Work out the finished part from the listing and answer in its coordinate system (mm). Face numbers are marked on the shaded views. A direction names the side the tool comes from. Round coordinates to 2 decimals unless told otherwise and drop trailing zeros. Loops run counter-clockwise (first coordinate to the right, second up) from the corner with the lowest first, then second, coordinate; pieces in that order, holes last. Notation, with made-up numbers: (58, -7.75) - (74, -7.75) arc R31 ccw to (74, 20.25) - close; hole circle Ø7 at (75, 38). An arc over 180 degrees is marked (long way). Use CSV: the item, a comma, the result in double quotes. Start each with the question number.
from build123d import *

# Parameters (mm, degrees)
F1_DEPTH = 20.32
F3_DEPTH = 15.24
F5_DEPTH = 25.4
F6_DEPTH = 3.175


with BuildPart() as f1:
    # F0 (on Front) → F1 (new body)
    with BuildSketch(Plane.XZ):
        Polygon((0, 31.623), (0, 0), (37.719, 0), (37.719, 3.175), (6.0198, 3.175), (6.0198, 31.623), align=None)
    extrude(amount=F1_DEPTH)

    # F2 (on face) → F3 (cut)
    with BuildSketch(Plane(origin=(0, 0, 0), x_dir=(1, 0, 0), z_dir=(0, 0, -1))):
        with BuildLine():
            Line((22.479, 6.858), (30.099, 6.858))
            ThreePointArc((30.099, 6.858), (33.401, 10.16), (30.099, 13.462))
            Line((30.099, 13.462), (22.479, 13.462))
            ThreePointArc((22.479, 13.462), (19.177, 10.16), (22.479, 6.858))
        make_face()
    extrude(amount=-F3_DEPTH, mode=Mode.SUBTRACT)

    # F4 (on face) → F5 (cut)
    with BuildSketch(Plane(origin=(0, 0, 0), x_dir=(0, -1, 0), z_dir=(-1, 0, 0))):
        with BuildLine():
            Line((13.462, 12.573), (13.462, 25.273))
            ThreePointArc((13.462, 25.273), (10.16, 28.575), (6.858, 25.273))
            Line((6.858, 25.273), (6.858, 12.573))
            ThreePointArc((6.858, 12.573), (10.16, 9.271), (13.462, 12.573))
        make_face()
    extrude(amount=-F5_DEPTH, mode=Mode.SUBTRACT)

    # F4 (on face) → F6 (cut)
    with BuildSketch(Plane(origin=(0, 0, 0), x_dir=(0, -1, 0), z_dir=(-1, 0, 0))):
        with BuildLine():
            Line((15.24, 12.573), (15.24, 25.273))
            ThreePointArc((15.24, 25.273), (10.16, 30.353), (5.08, 25.273))
            Line((5.08, 25.273), (5.08, 12.573))
            ThreePointArc((5.08, 12.573), (10.16, 7.493), (15.24, 12.573))
        make_face()
        with BuildLine():
            ThreePointArc((6.858, 25.273), (10.16, 28.575), (13.462, 25.273))
            Line((13.462, 25.273), (13.462, 12.573))
            ThreePointArc((13.462, 12.573), (10.16, 9.271), (6.858, 12.573))
            Line((6.858, 12.573), (6.858, 25.273))
        make_face(mode=Mode.SUBTRACT)
    extrude(amount=-F6_DEPTH, mode=Mode.SUBTRACT)


solid = f1.part
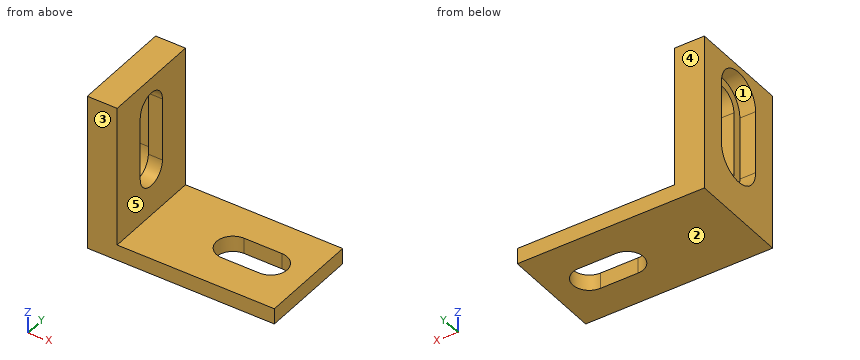
Item 1: Each of these flat-tipped pins is pushed along its axis until it touches: pin 1 Ø8 at (y, z) = (-9.5, 22.5) entering from +X; pin 2 Ø8 at (x, y) = (31, -12.5) entering from +Z (3 decimals). Where does it stop, or does it pass through?
Item 2: Find the intervals of material crossed by probe 1 along Y at (x, z) = (22.5, 3); probe 2 along Z at (x, y) = (15.5, -15.5) (3 decimals); probe 3 along X at (y, z) = (-5, 10), in increasing order. Write a range as [from, to].
Item 3: The mould has two halves that part along Y. Classify the marked faces 1, 2 and 3: pulls with the +Y half, pulls with the -Y half, needs draft (parallel to the pull), parting line crosses it, or undercut.
Item 4: Which of the six approach directions +Z, -Z, +X, -X, +Y, -Y give full straight-line access (tool end or side, diameter ignored) to the marked faces 4 and 5?
Item 5: A cutting plane is placed at B-B (z = 18.5). Determine the outline of the cut face in (x, y) (3 decimals), plus the area to 3 significant figures.
Item 6: A cutting plane is placed at C-C (y = -17.5). Determine the outline of the cut face in (x, z) (3 decimals), plus the area to 3 significant figures.
Item 7: A cutting plane is placed at A-A (y = -10.16). Determine the outline of the cut face in (x, z) (3 decimals), plus the area to 3 significant figures.
Item 8: A cutting plane is placed at D-D (z = 5.5). Determine the outline of the cut face in (x, y).
Result sheet:
1,pin 1,"x = 6.02"
1,pin 2,"z = 3.175"
2,probe 1,"[-20.32, -13.46], [-6.86, 0]"
2,probe 2,"[0, 3.175]"
2,probe 3,"[0, 6.02]"
3,face 1,"undercut"
3,face 2,"needs draft"
3,face 3,"pulls with the -Y half"
4,face 4,"+Z, -Z, +X, -X, +Y"
4,face 5,"+Z, +X, +Y, -Y"
5,outline,"(0, -20.32) - (6.02, -20.32) - (6.02, -13.462) - (3.175, -13.462) - (3.175, -15.24) - (0, -15.24) - close; (0, -5.08) - (3.175, -5.08) - (3.175, -6.858) - (6.02, -6.858) - (6.02, 0) - (0, 0) - close"
5,area,"71.3 mm^2"
6,outline,"(0, 0) - (37.719, 0) - (37.719, 3.175) - (6.02, 3.175) - (6.02, 31.623) - (0, 31.623) - close"
6,area,"291 mm^2"
7,outline,"(0, 0) - (19.177, 0) - (19.177, 3.175) - (6.02, 3.175) - (6.02, 9.271) - (3.175, 9.271) - (3.175, 7.493) - (0, 7.493) - close; (0, 30.353) - (3.175, 30.353) - (3.175, 28.575) - (6.02, 28.575) - (6.02, 31.623) - (0, 31.623) - close; (33.401, 0) - (37.719, 0) - (37.719, 3.175) - (33.401, 3.175) - close"
7,area,"118 mm^2"
8,outline,"(0, -20.32) - (6.02, -20.32) - (6.02, 0) - (0, 0) - close"
